Here's how the part is built. I have some questions about the finished solid (model axes, mm). Face numbers are marked on the shaded views. A direction names the side the tool comes from. Coordinates: 2 decimals unless noted, no trailing zeros. Write each loop counter-clockwise with the first axis right and the second up, starting at its lowest first coordinate (ties: lowest second). Pieces come first, ordered by that corner, then holes.
(1) For pin 1 Ø4 at (y, z) = (-91.5, -5.5) entering from -X; pin 2 Ø8 at (x, y) = (25, -124) entering from +Z; pin 3 Ø6 at (x, z) = (-48.5, 23) entering from -Y, each with a flat end and sliding along its axis, tell me the tip position at first contact or that it passes through.
(2) Which directions (+Z, -Z, +X, -X, +Y, -Y) give clear straight access to the entire face, cutting with the end or side of a thin tool? Please do the marked faces 1, 2 and 3.
(3) Thinking about a two-plate mould opening in X: for the marked faces 4, 5 and 6, which applies, released by +X, released by -X, zero draft, split by the parting line, or undercut?
(4) Please list where these lines run through material, in increasing order: probe 1 along Z at (x, y) = (0, 8.5); probe 2 along Y at (x, z) = (27, 56).
(5) Imagine slicing it at A-A, the plane y = -25.5. List the corners of the cut face in (x, z) for me (3 decimals), plus the area to 3 significant figures.
```python
from build123d import *

# Parameters (mm, degrees)
SKETCH1_R           = 63.5
SKETCH1_R_2         = 38.1
BOSS_EXTRUDE1_DEPTH = 25.4
FILLET1_R           = 5.08


with BuildPart() as part:
    # Sketch1 → Boss-Extrude1 (new body)
    with BuildSketch(Plane(origin=(0, 0, 0), x_dir=(1, 0, 0), z_dir=(0, 1, 0))):
        Circle(SKETCH1_R)
        Circle(SKETCH1_R_2, mode=Mode.SUBTRACT)
    extrude(amount=BOSS_EXTRUDE1_DEPTH)

    # Sketch4 → Revolve1 (revolve)
    with BuildSketch(Plane.XY):
        Polygon((50.8, 0), (12.7, -76.2), (6.35, -76.2), (38.1, 0), align=None)
    revolve(axis=Axis((0, -76.2, 0), (0, 1, 0)))

    # Sketch6 → Revolve2 (revolve)
    with BuildSketch(Plane.XY):
        Polygon((12.7, -76.2), (38.1, -152.4), (25.4, -152.4), (6.35, -76.2), align=None)
    revolve(axis=Axis((0, -76.2, 0), (0, -1, 0)))

    # Fillet1
    fillet1_edges = [part.edges().sort_by_distance(p)[0] for p in [
        (-6.35, -76.2, 0),
    ]]
    fillet(fillet1_edges, radius=FILLET1_R)


solid = part.part
```
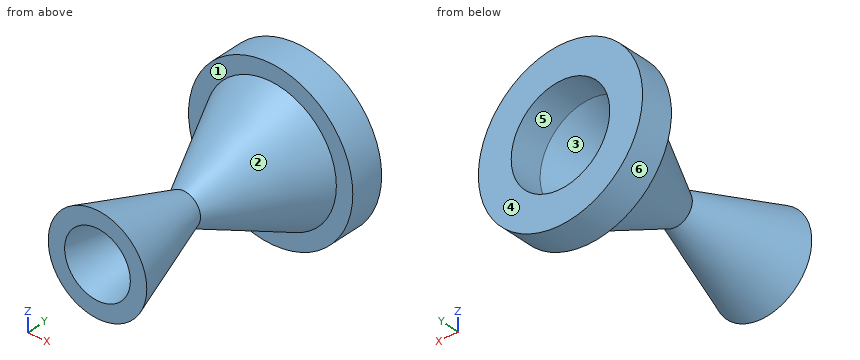
Recorded:
1. pin 1: stops at x = -17.82
1. pin 2: stops at z = 19.89
1. pin 3: stops at y = -0.25
2. face 1: -Y
2. face 2: none
2. face 3: +Y
3. face 4: zero draft
3. face 5: undercut
3. face 6: split by the parting line
4. probe 1: z = -63.5 to -38.1, 38.1 to 63.5
4. probe 2: y = 0 to 25.4
5. outline: circle Ø76.1 at (0, 0); hole circle Ø54.95 at (0, 0)
5. area: 2,180 mm2
